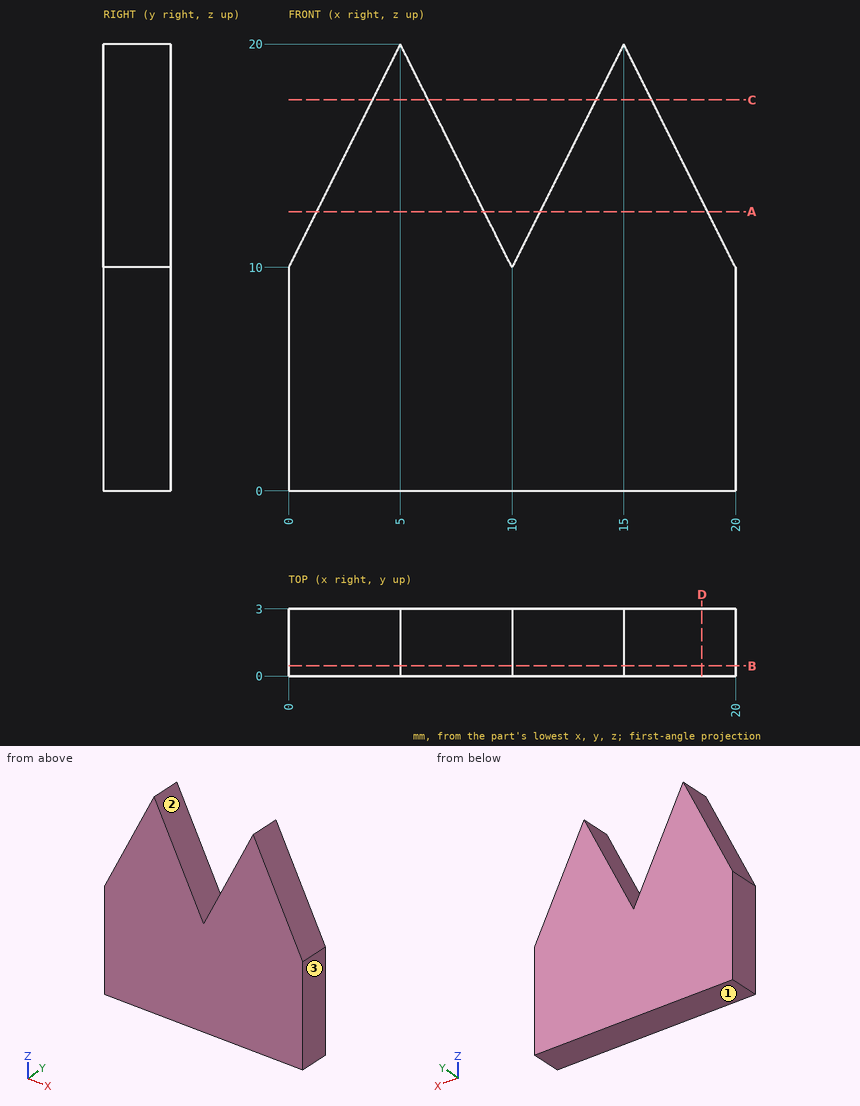
Answer from the drawing. Dimensions are ordinates in mm from the lowest x, y and z of the part. Round coordinates to 2 decimals unless told otherwise and drop trailing zeros. Loops run counter-clockwise (first coordinate to the right, second up) from the corner with the lowest first, then second, coordinate; pieces in that order, holes last. Notation, with made-up numbers: (5.25, 9.5) - (64.25, 9.5) arc R26 cw to (64.25, 36.5) - close; hole circle Ø10 at (72, 66). An arc over 180 degrees is marked (long way). Return JSON: item names as keys, results as strings. Group by question number.
1. The part is cut by section D-D on x = 18.5. Determine the outline of the cut face in (y, z), then the cut area to 3 significant figures.
2. The part is cut by section A-A on z = 12.5. Determine the outline of the cut face in (x, y).
3. This flat-tipped pin is pushed along its axis until it touches: P1, Ø1, axis at y = 0.5, z = 11, coming from the -X side. Where does it stop, or does it pass through?
4. The part is cut by section C-C on z = 17.5. Determine the outline of the cut face in (x, y).
5. The mould has two halves that part along X. Classify the marked faces 1, 2 and 3: pulls with the +X half, pulls with the -X half, needs draft (parallel to the pull), parting line crosses it, or undercut.
6. The part is cut by section B-B on y = 0.45. Determine the outline of the cut face in (x, z).
7. Consider probe 1 along X at (y, z) = (0.3, 16.5); probe 2 along X at (y, z) = (2.8, 13); probe 3 along Z at (x, y) = (12.5, 0.9). Determine where each line is inside the solid, lowest interval first.
Resolved:
{
 "1": {"outline": "(0, 0) - (3, 0) - (3, 13) - (0, 13) - close", "area": "39.0 mm²"},
 "2": {"outline": "(1.25, 0) - (8.75, 0) - (8.75, 3) - (1.25, 3) - close; (11.25, 0) - (18.75, 0) - (18.75, 3) - (11.25, 3) - close"},
 "3": {"P1": "stops at x = 0.25"},
 "4": {"outline": "(3.75, 0) - (6.25, 0) - (6.25, 3) - (3.75, 3) - close; (13.75, 0) - (16.25, 0) - (16.25, 3) - (13.75, 3) - close"},
 "5": {"face 1": "needs draft", "face 2": "undercut", "face 3": "pulls with the +X half"},
 "6": {"outline": "(0, 0) - (20, 0) - (20, 10) - (15, 20) - (10, 10) - (5, 20) - (0, 10) - close"},
 "7": {"probe 1": "x = 3.25 to 6.75, 13.25 to 16.75", "probe 2": "x = 1.5 to 8.5, 11.5 to 18.5", "probe 3": "z = 0 to 15"}
}
